Check sheet for the modelled part. Datum: model origin and axes. Units: mm. Face numbers are marked on the shaded views. Coordinates: 2 decimals unless noted, no trailing zeros.
1. Thickness scan on line 1 (Z direction, x = 58.5, y = -7); line 2 (X direction, y = -64, z = 38); line 3 (Z direction, x = 36.5, y = 7). Record the ranges inside material, lowest first.
2. Draft check along Z on the marked faces 1 and 2. Enter one of: released by +Z, released by -Z, zero draft, split by the parting line, or undercut.
3. Gauge pin test, flat ends, axial feed: pin 1 Ø2 at (x, z) = (54.5, -10) entering from -Y; pin 2 Ø4.5 at (y, z) = (14.732, 0) entering from +X; pin 3 Ø5 at (y, z) = (72, -22) entering from -X; pin 4 Ø5.5 at (x, y) = (-75, -0.5) entering from +Z. Record the tip position at first contact, or that the pin passes through.
```python
from build123d import *

# Parameters (mm, degrees)
BOSS_EXTRUDE1_START = -11.43
BOSS_EXTRUDE1_DEPTH = 22.86
SKETCH3_R           = 2.38125
CUT_EXTRUDE1_DEPTH  = 239.515332253
CIRPATTERN1_COUNT   = 4
BOSS_EXTRUDE2_DEPTH = 6.35


with BuildPart() as part:
    # Sketch1 → Revolve1 (revolve)
    with BuildSketch(Plane.XY, mode=Mode.PRIVATE) as revolve1_sk:
        with BuildLine():
            Line((0, 165.1), (0, 162.1028))
            add(Edge.make_bspline(
                [(79.315278355, 1.342862767), (78.663627327, 162.1028), (0, 162.1028)],
                knots=[4.720673095, 4.720673095, 4.720673095, 6.283185307, 6.283185307, 6.283185307], degree=2, weights=[1, 0.710029584, 1]))
            Line((79.315278355, 1.342862767), (77.575, -0.397415588))
            Line((77.575, -0.397415588), (77.575, -80.518))
            Line((77.575, -80.518), (79.375, -80.518))
            Line((79.375, -80.518), (79.375, -1.143))
            Line((79.375, -1.143), (80.518, 0))
            add(Edge.make_bspline(
                [(80.518, 0), (80.518, 165.1), (0, 165.1)],
                knots=[1.570796327, 1.570796327, 1.570796327, 3.141592654, 3.141592654, 3.141592654], degree=2, weights=[1, 0.707106781, 1]))
        make_face()
    revolve(revolve1_sk.sketch.rotate(Axis((0, 165.1, 0), (0, -1, 0)), 90), axis=Axis((0, 165.1, 0), (0, -1, 0)))

    # Sketch6 → Boss-Extrude1 (add)
    with BuildSketch(Plane.XY.offset(BOSS_EXTRUDE1_START)):
        with BuildLine():
            Line((73.66, 21.470281301), (78.034242777, 29.046692038))
            add(Edge.make_bspline(
                [(79.062314745, 13.005354783), (78.744364926, 21.078512305), (78.034242777, 29.046692038)],
                knots=[4.792704356, 4.792704356, 4.792704356, 4.892548854, 4.892548854, 4.892548854], degree=2, weights=[1, 0.998754143, 1]))
            add(Edge.make_bspline(
                [(79.315278355, 1.342862767), (79.29160326, 7.183422549), (79.062314745, 13.005354783)],
                knots=[4.720673095, 4.720673095, 4.720673095, 4.792704356, 4.792704356, 4.792704356], degree=2, weights=[1, 0.999351507, 1]))
            Line((79.315278355, 1.342862767), (77.575, -0.397415588))
            Line((77.575, -0.397415588), (77.575, -18.537382644))
            Line((77.575, -18.537382644), (73.66, -11.756403732))
            Line((73.66, -11.756403732), (73.66, 17.13351746))
            Line((73.66, 17.13351746), (73.66, 21.470281301))
        make_face()
    boss_extrude1 = extrude(amount=BOSS_EXTRUDE1_DEPTH)

    # Sketch3 → Cut-Extrude1 (cut, through all)
    with BuildSketch(Plane.ZY.offset(-71.628)):
        with Locations(Location((0, 14.732, 0), (0, 0, 270))):
            Circle(SKETCH3_R)
    cut_extrude1 = extrude(amount=-CUT_EXTRUDE1_DEPTH, mode=Mode.SUBTRACT)

    # CirPattern1: Boss-Extrude1, Cut-Extrude1 ×4 about axis
    cirpattern1_axis = Axis((0, 0, 0), (0, 1, 0))
    add([boss_extrude1.rotate(cirpattern1_axis, i * 360 / CIRPATTERN1_COUNT) for i in range(1, CIRPATTERN1_COUNT)])
    add([cut_extrude1.rotate(cirpattern1_axis, i * 360 / CIRPATTERN1_COUNT) for i in range(1, CIRPATTERN1_COUNT)], mode=Mode.SUBTRACT)

    # Sketch7 → Boss-Extrude2 (add, symmetric)
    with BuildSketch(Plane(origin=(0, -74.168, 0), x_dir=(1, 0, 0), z_dir=(0, 0, 1))):
        with BuildLine():
            Line((73.66, 95.638281301), (78.034242777, 103.214692038))
            add(Edge.make_bspline(
                [(78.034242777, 103.214692038), (76.413302416, 121.403033529), (72.830065055, 138.378377261)],
                knots=[1.750956201, 1.750956201, 1.750956201, 1.978071652, 1.978071652, 1.978071652], degree=2, weights=[1, 0.993559247, 1]))
            Line((72.830065055, 138.378377261), (73.66, 95.638281301))
        make_face()
    extrude(amount=BOSS_EXTRUDE2_DEPTH, both=True)


solid = part.part
```
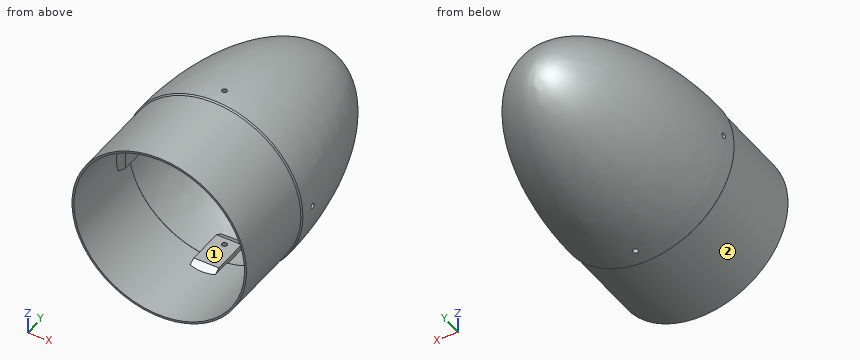
Data:
1. line 1: z = -53.65 to -50.95, 50.95 to 53.65
1. line 2: x = -69.69 to -67.63, 67.63 to 69.69
1. line 3: z = -71.69 to -70.34, 70.34 to 71.69
2. face 1: undercut
2. face 2: split by the parting line
3. pin 1: stops at y = 113.96
3. pin 2: passes through
3. pin 3: stops at x = -70.01
3. pin 4: stops at z = 35.45
